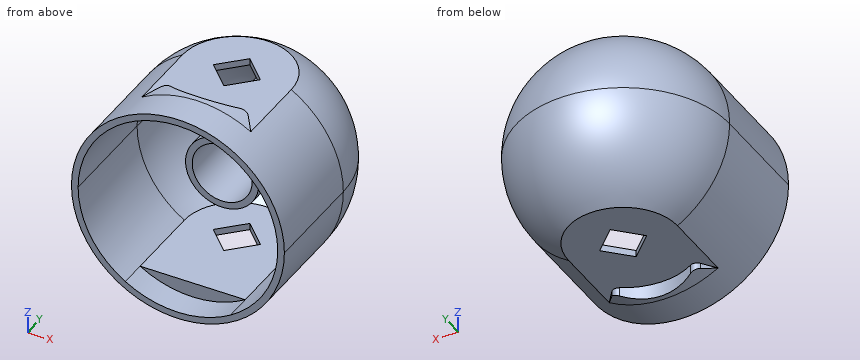
from build123d import *

# Parameters (mm, degrees)
REVOLVE1_ANGLE           = 180
CUT_EXTRUDE1_DEPTH       = 39.328351126
SHELL1_DEPTH             = 16
SHELL1_2_DEPTH           = 4
EXTRUDE1_REACH           = 40.328
EXTRUDE1_END_RADIUS      = 16
CUT_EXTRUDE2_REACH       = 40.328
EXTRUDE_THIN1_REACH      = 53.192
EXTRUDE_THIN1_END_RADIUS = 15
EXTRUDE_THIN1_START      = -12
SKETCH5_R                = 5.5
SKETCH5_R_2              = 4.5
FILLET_1_R               = 1


with BuildPart() as part:
    # Sketch1 → Revolve1 (revolve)
    with BuildSketch(Plane(origin=(0, 0, 0), x_dir=(-1, 0, 0), z_dir=(0, 0, -1))):
        with BuildLine():
            Line((0, 0), (16, 0))
            Line((16, 0), (16, 16))
            ThreePointArc((16, 16), (11.313708499, 27.313708499), (0, 32))
            Line((0, 32), (0, 0))
        make_face()
    revolve(axis=Axis((0, 0, 0), (0, 1, 0)), revolution_arc=REVOLVE1_ANGLE)

    # Sketch2 → Cut-Extrude1 (cut, through all)
    with BuildSketch(Plane.XY.offset(13.75)):
        with BuildLine():
            Line((8.181534086, 5), (8.181534086, 16))
            ThreePointArc((8.181534086, 16), (0, 24.181534086), (-8.181534086, 16))
            Line((-8.181534086, 16), (-8.181534086, 5))
            Line((-8.181534086, 5), (8.181534086, 5))
        make_face()
    extrude(amount=CUT_EXTRUDE1_DEPTH, mode=Mode.SUBTRACT)

    # Shell1: read off the stored shape, not the designer's step
    # Shell1 outline → Shell1 (cut)
    with BuildSketch(Plane(origin=(0, 0, 0), x_dir=(1, 0, 0), z_dir=(0, 1, 0))):
        with BuildLine():
            ThreePointArc((7.901740315, -12.75), (13.105840391, -7.296365372), (15, 0))
            Line((15, 0), (-15, 0))
            ThreePointArc((-15, 0), (-13.105840391, -7.296365372), (-7.901740315, -12.75))
            Line((-7.901740315, -12.75), (7.901740315, -12.75))
        make_face()
    extrude(amount=SHELL1_DEPTH, mode=Mode.SUBTRACT)

    # Shell1 2 outline → Shell1 2 (cut)
    with BuildSketch(Plane(origin=(0, 0, 0), x_dir=(1, 0, 0), z_dir=(0, 1, 0))):
        with BuildLine():
            ThreePointArc((-7.901740315, -12.75), (0, -15), (7.901740315, -12.75))
            Line((7.901740315, -12.75), (-7.901740315, -12.75))
        make_face()
    extrude(amount=SHELL1_2_DEPTH, mode=Mode.SUBTRACT)

    # Shell1 3 outline → Shell1 3 (revolve, cut)
    with BuildSketch(Plane.XZ.offset(-16)):
        with BuildLine():
            ThreePointArc((15, 0), (13.105840391, 7.296365372), (7.901740315, 12.75))
            Line((7.901740315, 12.75), (0, 12.75))
            Line((0, 12.75), (0, 0))
            Line((0, 0), (15, 0))
        make_face()
    revolve(axis=Axis((0, 16, 0), (0, 0, 1)), mode=Mode.SUBTRACT)

    # Extrude1: up to this cylinder (the profile starts inside it)
    extrude1_end = Plane(origin=(0, 6.31611, 0), z_dir=(0, -1, 0)) * Cylinder(EXTRUDE1_END_RADIUS, 113.656, mode=Mode.PRIVATE)
    # Sketch3 → Extrude1 (add, up to the surface)
    with BuildSketch(Plane.XY.offset(13.75), mode=Mode.PRIVATE) as extrude1_sk1:
        with BuildLine():
            Line((6.076328446, 7.830430308), (8.181534086, 5))
            Line((8.181534086, 5), (-8.181534086, 5))
            Line((-8.181534086, 5), (-6.076328446, 7.830430308))
            ThreePointArc((-6.076328446, 7.830430308), (0, 5.818465914), (6.076328446, 7.830430308))
        make_face()
    extrude1_tool1 = extrude(extrude1_sk1.sketch, amount=EXTRUDE1_REACH, mode=Mode.PRIVATE) & extrude1_end
    add(extrude1_tool1.solids().sort_by_distance((6.995686, 6.31611, 13.75))[0])

    # Sketch4 → Cut-Extrude2 (cut, up to next)
    with BuildSketch(Plane.XY.offset(13.75), mode=Mode.PRIVATE) as cut_extrude2_sk1:
        Polygon((-3.535533906, 16), (0, 12.464466094), (3.535533906, 16), (0, 19.535533906), align=None)
    cut_extrude2_tool1 = extrude(cut_extrude2_sk1.sketch, amount=-CUT_EXTRUDE2_REACH, mode=Mode.PRIVATE) & part.part
    add(cut_extrude2_tool1.solids().sort_by_distance((0, 16, 13.75))[0], mode=Mode.SUBTRACT)

    # Mirror1: part across face


with BuildPart() as part_1:
    add(part.part)
    add(part.part.mirror(Plane(origin=(0, 18.784156894, 0), x_dir=(1, 0, 0), z_dir=(0, 0, -1))))

    # Extrude-Thin1: up to this sphere (the profile starts inside it)
    extrude_thin1_end = Location((0, 16, 0)) * Sphere(EXTRUDE_THIN1_END_RADIUS, mode=Mode.PRIVATE)
    # Sketch5 → Extrude-Thin1 (add, up to the surface)
    with BuildSketch(Plane.XZ.offset(EXTRUDE_THIN1_START), mode=Mode.PRIVATE) as extrude_thin1_sk1:
        Circle(SKETCH5_R)
        Circle(SKETCH5_R_2, mode=Mode.SUBTRACT)
    extrude_thin1_tool1 = extrude(extrude_thin1_sk1.sketch, amount=-EXTRUDE_THIN1_REACH, mode=Mode.PRIVATE) & extrude_thin1_end
    add(extrude_thin1_tool1.solids().sort_by_distance((-5.344437, 12, 0))[0])

    # 圓角1
    fillet_1_edges = [part_1.edges().sort_by_distance(p)[0] for p in [
        (6.076328446, 7.830430308, 14.275645793),
        (-6.076328446, 7.830430308, 14.275645793),
        (-6.076328446, 7.830430308, -14.275645793),
        (6.076328446, 7.830430308, -14.275645793),
    ]]
    fillet(fillet_1_edges, radius=FILLET_1_R)


solid = part_1.part
Here's how the part is built. I have some questions about the finished solid (model axes, mm). Round coordinates to 2 decimals unless told otherwise and drop trailing zeros. Loops run counter-clockwise (first coordinate to the right, second up) from the corner with the lowest first, then second, coordinate; pieces in that order, holes last.
1. If we section it at C-C on x = 12: Write out the boundary of the cut face in (y, z), plus the area to 3 significant figures.
Answer list:
outline: (0, -10.58) - (16, -10.58) arc R10.58 ccw to (16, 10.58) - (0, 10.58) - (0, 9) - (16, 9) arc R9 cw to (16, -9) - (0, -9) - close
area: 99.4 mm2
2. If I drill on line 1 along Z through (x, y) = (0, 20); line 2 along Z through (x, y) = (1.5, 8.5); line 3 along Z through (x, y) = (-2, 26), over which ranges is the centre line in solid material (lowest first)?
Answer list:
line 1: z = -13.75 to -12.75, -5.5 to -4.5, 4.5 to 5.5, 12.75 to 13.75
line 2: z = -13.75 to -12.75, 12.75 to 13.75
line 3: z = -12.33 to -11, -5.12 to -4.03, 4.03 to 5.12, 11 to 12.33
3. If we section it at A-A on y = 21: Write out the boundary of the cut face in (x, z), plus the area to 3 significant figures.
Answer list:
outline: (-6.48, -13.75) - (6.48, -13.75) arc R15.2 ccw to (6.48, 13.75) - (-6.48, 13.75) arc R15.2 ccw to start; circle Ø11 at (0, 0); hole (-6.12, -12.75) - (6.12, -12.75) arc R14.14 ccw to (6.12, 12.75) - (-6.12, 12.75) arc R14.14 ccw to start; hole circle Ø9 at (0, 0)
area: 126 mm2
4. If we section it at D-D on z = -5: Write out the boundary of the cut face in (x, y), plus the area to 3 significant figures.
Answer list:
outline: (-15.2, 0) - (-14.14, 0) - (-14.14, 16) arc R14.14 cw to (-2.29, 29.96) - (-2.29, 12) - (2.29, 12) - (2.29, 29.96) arc R14.14 cw to (14.14, 16) - (14.14, 0) - (15.2, 0) - (15.2, 16) arc R15.2 ccw to (-15.2, 16) - close
area: 165 mm2
5. For P1, Ø1.1, axis at x = 1.5, z = -13.5, coming from the -Y side; P2, Ø5, axis at x = 8.5, y = 16, coming from the +Z side; P3, Ø2, axis at x = -5.5, y = 23.5, coming from the +Z side, each with a flat end and sliding along its axis, tell me the tip position at first contact or that it passes through.
Answer list:
P1: stops at y = 4
P2: stops at z = 13.75
P3: stops at z = 13.68
6. If we section it at B-B on y = 10: Write out the boundary of the cut face in (x, z).
Answer list:
outline: (-8.18, -13.75) - (8.18, -13.75) arc R16 ccw to (8.18, 13.75) - (-8.18, 13.75) arc R16 ccw to start; hole (-7.9, -12.75) - (7.9, -12.75) arc R15 ccw to (7.9, 12.75) - (-7.9, 12.75) arc R15 ccw to start
